```python
from build123d import *

# Parameters (mm, degrees)
SKETCH1_R                        = 6.35
BOSS_EXTRUDE1_DEPTH              = 25.4
SKETCH3_R                        = 4.7625
CUT_EXTRUDE1_DEPTH               = 27.940768363
F_1_8_0_125_DIAMETER_HOLE2_D     = 3.175
F_1_8_0_125_DIAMETER_HOLE2_DEPTH = 6.349
F_1_8_0_125_DIAMETER_HOLE2_TIP   = 0.953866233


with BuildPart() as part:
    # Sketch1 → Boss-Extrude1 (new body)
    with BuildSketch(Plane(origin=(0, 0, 0), x_dir=(1, 0, 0), z_dir=(0, 1, 0))):
        with Locations(Location((0, 0, 0), (0, 0, 270))):
            Circle(SKETCH1_R)
    extrude(amount=BOSS_EXTRUDE1_DEPTH)

    # Sketch3 → Cut-Extrude1 (cut, through all)
    with BuildSketch(Plane(origin=(0, 25.4, 0), x_dir=(1, 0, 0), z_dir=(0, 1, 0))):
        with Locations(Location((0, 0, 0), (0, 0, 270))):
            Circle(SKETCH3_R)
    extrude(amount=-CUT_EXTRUDE1_DEPTH, mode=Mode.SUBTRACT)

    # 1/8 (0.125) Diameter Hole2
    with Locations(Plane(origin=(-0.004002873, 6.346663359, 6.349998738), x_dir=(0.999999801314, 0, 0.000630373746), z_dir=(-0.000630373746, 0, 0.999999801314))):
        with Locations((0, 0)):
            Hole(F_1_8_0_125_DIAMETER_HOLE2_D / 2, depth=F_1_8_0_125_DIAMETER_HOLE2_DEPTH)
            with Locations((0, 0, -(F_1_8_0_125_DIAMETER_HOLE2_DEPTH + F_1_8_0_125_DIAMETER_HOLE2_TIP / 2))):  # 118° drill point
                Cone(0, F_1_8_0_125_DIAMETER_HOLE2_D / 2, F_1_8_0_125_DIAMETER_HOLE2_TIP, mode=Mode.SUBTRACT)


solid = part.part
```
Could you check a few things on this model? Use its own coordinates, in mm. Coordinates: 2 decimals unless noted, no trailing zeros. Loops run counter-clockwise (first coordinate to the right, second up) from the corner with the lowest first, then second, coordinate; pieces in that order, holes last.
1) Thinking about a two-plate mould opening in Z: for faces 1 (the face through (5, 25.4, 1)), 2 (the face through (-2.9, 12.88, -3.78)), 3 (the face through (-3.86, 12.52, -5.04)), which applies, released by +Z, released by -Z, zero draft, split by the parting line, or undercut?
Reported:
face 1: zero draft
face 2: undercut
face 3: split by the parting line
2) Imagine slicing it at A-A (z = 0). List the corners of the cut face in (x, y) for me.
Reported:
outline: (-6.35, 0) - (-4.76, 0) - (-4.76, 25.4) - (-6.35, 25.4) - close; (4.76, 0) - (6.35, 0) - (6.35, 25.4) - (4.76, 25.4) - close
3) Please list where these lines run through material, in increasing order: line 1 along X through (y, z) = (10, 0); line 2 along Z through (x, y) = (-3.5, 19); line 3 along X through (y, z) = (14.75, -2).
Reported:
line 1: x = -6.35 to -4.76, 4.76 to 6.35
line 2: z = -5.3 to -3.23, 3.23 to 5.3
line 3: x = -6.03 to -4.32, 4.32 to 6.03
4) Imagine slicing it at B-B (x = 0). State how many separate pieces and enclosed holes the cut face has, and give its area (3 significant figures).
Reported:
separate pieces: 3
enclosed holes: 0
area: 75.6 mm2
5) Imagine slicing it at D-D (x = -2). List the corners of the cut face in (y, z) for me, and give its area (3 significant figures).
Reported:
outline: (0, -6.03) - (25.4, -6.03) - (25.4, -4.32) - (0, -4.32) - close; (0, 4.32) - (25.4, 4.32) - (25.4, 6.03) - (0, 6.03) - close
area: 86.6 mm2
6) Will these pins go through, and if not, where does the flat tip stop? pin 1 Ø1.5 at (x, y) = (2.5, 3) entering from +Z; pin 2 Ø1.5 at (y, z) = (14, 3) entering from -X; pin 3 Ø1 at (y, z) = (23, -4.5) entering from +X.
Reported:
pin 1: stops at z = 6.1
pin 2: stops at x = -5.94
pin 3: stops at x = 4.93
